Can you work these out from the model? Positions are in its coordinate system, mm. Face numbers are marked on the shaded views. A direction names the side the tool comes from. Coordinates: 2 decimals unless noted, no trailing zeros. Write each loop counter-clockwise with the first axis right and the second up, starting at its lowest first coordinate (ties: lowest second). Pieces come first, ordered by that corner, then holes.
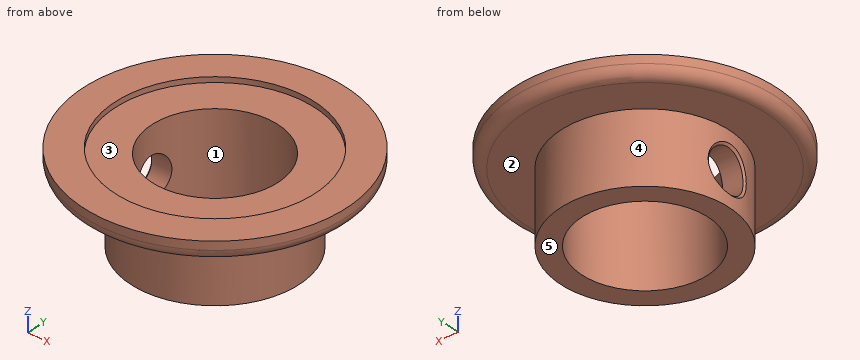
Autodesk Inventor part; units mm, degrees
ref_plane "YZ Plane" through (0, 0, 0) normal (1, 0, 0) x (0, 1, 0)
ref_plane "XZ Plane" through (0, 0, 0) normal (0, 1, 0) x (-1, 0, 0)
ref_plane "XY Plane" through (0, 0, 0) normal (0, 0, 1) x (1, 0, 0)
sketch "Sketch1" plane through (0, 0, 0) normal (1, 0, 0) x (0, 1, 0)
  line L0 (6, 3) -> (6, -3)
  line L1 (8, 1.7) -> (11.5, 1.7)
  line L2 (12.5, 2.7) -> (12.5, 3.5)
  line L3 (12.5, 2.7) -> (11.5, 2.7) construction
  line L4 (11.5, 2.7) -> (11.5, 1.7) construction
  arc A0 (11.5, 1.7) -> (12.5, 2.7) centre (11.5, 2.7) ccw
  line L5 (6, 3) -> (9.5, 3)
  line L6 (12.5, 3.5) -> (9.5, 3.5)
  line L7 (9.5, 3.5) -> (9.5, 3)
  line L8 (0, 0) -> (0, 11.4482) construction
  line L9 (8, -3) -> (8, 1.7)
  line L10 (6, -3) -> (6, -5)
  line L11 (6, -5) -> (8, -5)
  line L12 (8, -5) -> (8, -3)
  point P0 (7, 0.2)
  dimension "d0" = 6
  dimension "d1" = 3
  dimension "d5" = 0.8
  dimension "d6" = 1
  dimension "d7" = 1
  dimension "d8" = 3
  dimension "d10" = 6
  dimension "d12" = 0.5
  dimension "d14" = 3.5
  dimension "d26" = 2
  dimension "d27" = 4.7
revolve "Revolution1" add sketch "Sketch1" angle 360 about axis through (0, 0, 0) along (0, 0, 1)
ref_plane "Work Plane2" through (-7.9989, -0.1297, -1.65) normal (-0.9998686, -0.0162116, 0) x (0, 0, 1)
ref_plane "Work Plane1" through (21.3966, -11.9547, -30.348) normal (-0.9998686, -0.0162116, 0) x (0, 0, 1)
sketch "Sketch2" plane through (-7.9989, -0.1297, -1.65) normal (-0.9998686, -0.0162116, 0) x (0, 0, 1)
  circle A0 centre (0, 0) radius 1.5
  point P0 (1.65, 0)
  dimension "d15" = 3
hole "Hole1" at (-7.9989, -0.1297, -1.65) direction (0.9998686, 0.0162116, 0) diameter 4 depth 8.8 tip angle 118
chamfer "Chamfer1" distance 0.2 angle 45 2 edges at (-7.8033, 1.7632, -0.9945) (-7.742, -2.0152, -0.9943)
ref_plane "Work Plane4" through (-7.9989, -0.1297, 0.55) normal (-0.9998686, -0.0162116, 0) x (0.0162116, -0.9998686, 0)
equation "\"d1\" = 0.5 * d0"
equation "\"d7\" = d6"
properties part number "tarcza sprzęgła"
1. If I drill on L1, parallel to X at y = 0, z = 3.4; L2, parallel to Y at x = 0, z = 0, over which ranges is the centre line in solid material (lowest first)?
2. We'd pull the mould along X, two halves only. Please class the marked faces 3, 4 and 5: released by +X, released by -X, zero draft, split by the parting line, or undercut.
3. If we section it at A-A, the plane x = 0: List the corners of the cut face in (y, z) for me, plus the area to 3 significant figures.
4. I'm going to push flat-ended pins straight in: P1, Ø5.5, axis at x = 2.5, y = -3, coming from the +Z side; P2, Ø3, axis at x = 4, z = -1, coming from the +Y side; P3, Ø1, axis at x = 5, y = 9, coming from the -Z side. Where does each tip first touch, or does it pass through?
5. If we section it at B-B, the plane y = 0.75: Count the separate pieces of the cut face and the enclosed holes in it, plus the area to 3 significant figures.
6. Which directions (+Z, -Z, +X, -X, +Y, -Y) give clear straight access to the entire face, cutting with the end or side of a thin tool? Please do the marked faces 1 and 2.
Answers:
1. L1: x = -12.5 to -9.5, 9.5 to 12.5
1. L2: y = -8 to -6, 6 to 8
2. face 3: undercut
2. face 4: split by the parting line
2. face 5: zero draft
3. outline: (-12.5, 2.7) arc R1 ccw to (-11.5, 1.7) - (-8, 1.7) - (-8, -5) - (-6, -5) - (-6, 3) - (-9.5, 3) - (-9.5, 3.5) - (-12.5, 3.5) - close; (6, -5) - (8, -5) - (8, 1.7) - (11.5, 1.7) arc R1 ccw to (12.5, 2.7) - (12.5, 3.5) - (9.5, 3.5) - (9.5, 3) - (6, 3) - close
3. area: 46.3 mm2
4. P1: stops at z = 3
4. P2: stops at y = 7.6
4. P3: stops at z = 1.7
5. separate pieces: 3
5. enclosed holes: 0
5. area: 39.2 mm2
6. face 1: +Z, -Z
6. face 2: -Z
